Autodesk Inventor part; units mm, degrees
ref_plane "YZ Plane" through (0, 0, 0) normal (1, 0, 0) x (0, 1, 0)
ref_plane "XZ Plane" through (0, 0, 0) normal (0, 1, 0) x (-1, 0, 0)
ref_plane "XY Plane" through (0, 0, 0) normal (0, 0, 1) x (1, 0, 0)
ref_plane "Work Plane1" through (0, 0, 0) normal (0, 0, 1) x (1, 0, 0)
sketch "Sketch1" plane through (0, 0, 0) normal (0, 0, 1) x (1, 0, 0)
  circle A0 centre (23.85, -37.9212) radius 0.7
  circle A1 centre (23.85, -26.8413) radius 0.7
  circle A2 centre (10.55, -52.3871) radius 14
  circle A3 centre (10.55, -11.45) radius 14
  line L0 (25.25, -34.8579) -> (25.25, -62.5871)
  line L1 (22.15, -44.5487) -> (26.25, -44.5487)
  line L2 (26.25, -44.5487) -> (26.25, -19.2884)
  line L3 (26.25, -19.2884) -> (22.15, -19.2884)
  line L4 (22.15, -19.2884) -> (22.15, -44.5487)
  circle A4 centre (24.2, -42.4987) radius 2.05
  circle A5 centre (24.2, -21.3384) radius 2.05
  point P0 (0, 0)
  point P1 (24.2, -19.2884)
  point P2 (22.15, -21.3384)
  point P3 (22.15, -42.4987)
  point P4 (24.2, -44.5487)
  dimension "d0" = 1
  dimension "d1" = 1
extrude "Extrusion1" add sketch "Sketch1" along normal blind 3.5 contours A0 | A1 | A4 L0 L1 | A4 L0 | L4 A5 L2 A4 | L0 A4 L2 L1 | L0 A4 | A5 | L3 L2 A5
sketch "Sketch2" plane through (0, 0, 3.5) normal (0, 0, 1) x (1, 0, 0)
  line L0 (22.25, -33.4185) -> (19.55, -33.4185)
  line L1 (22.25, -30.4185) -> (19.55, -30.4185)
  line L2 (26.25, -33.9066) -> (26.25, -41.9871)
  line L3 (26.25, -29.1685) -> (26.25, -34.6685)
  line L4 (26.25, -21.85) -> (26.25, -29.9304)
  line L5 (22.15, -21.3384) -> (22.15, -42.4987)
  line L6 (26.25, -33.9185) -> (20.65, -33.9185)
  line L7 (20.65, -33.9185) -> (20.65, -29.9185)
  line L8 (20.65, -29.9185) -> (26.25, -29.9185)
  line L9 (26.25, -29.9185) -> (26.25, -33.9185)
  point P0 (0, 0)
  dimension "d4" = 0.5
  dimension "d5" = 0.5
  dimension "d6" = 1.5
extrude "Extrusion2" add sketch "Sketch2" along normal blind 5.5
sketch "Sketch3" plane through (20.65, -33.9185, 3.5) normal (0, -1, 0) x (1, 0, 0)
  circle A0 centre (-2.1, 3) radius 1.25
  line L0 (5.6, 0) -> (5.6, 5.5)
  circle A1 centre (2.4, 3) radius 1.25
  line L1 (2.4, 3) -> (-2.1, 3)
  circle A2 centre (2.4, 3) radius 2.5
  point P0 (-20.65, -3.5)
  dimension "d17" = 5
  dimension "d18" = 0.7
extrude "Extrusion3" cut sketch "Sketch3" against normal blind 11.5 contours A1
fillet "Fillet1" radius 2 2 edges at (20.65, -31.9185, 9) (20.65, -31.9185, 3.5)
ref_plane "Work Plane2" through (0, 0, 19.2) normal (0, 0, 1) x (1, 0, 0)
mirror "Mirror1" about plane through (0, 0, 19.2) normal (0, 0, 1) of "Extrusion1", "Extrusion2", "Extrusion3", "Fillet1"
sketch "Sketch4" plane through (0, 0, 3.5) normal (0, 0, 1) x (1, 0, 0)
  line L0 (26.25, -44.5487) -> (26.25, -19.2884)
  line L1 (24.2, -44.5487) -> (26.25, -44.5487)
  line L2 (26.25, -19.2884) -> (24.2, -19.2884)
  line L3 (25.75, -44.5487) -> (25.75, -19.2884)
  arc A0 (22.15, -42.4987) -> (24.2, -44.5487) centre (24.2, -42.4987) ccw
  line L4 (22.15, -21.3384) -> (22.15, -42.4987)
  arc A1 (24.2, -19.2884) -> (22.15, -21.3384) centre (24.2, -21.3384) ccw
  line L5 (25.75, -40.5487) -> (22.15, -40.5487)
  point P0 (0, 0)
  dimension "d14" = 0.5
  dimension "d20" = 4
extrude "Extrusion4" add sketch "Sketch4" along normal up to surface (31.4 mm away) contours L1 L3 L2 L0 | L1 A0 L4 L5 L3
fillet "Fillet2" radius 0.5 7 edges at (25.75, -37.2336, 3.5) (25.75, -24.6035, 3.5) (25.75, -37.2336, 34.9) (25.75, -24.6035, 34.9) (25.75, -40.5487, 19.2) (25.75, -31.9185, 9) (25.75, -31.9185, 29.4)
sketch "Sketch5" plane through (24.2, -19.2884, 38.4) normal (0, 0, 1) x (1, 0, 0)
  circle A0 centre (-0.35, -17.7307) radius 0.7
  circle A1 centre (-0.35, -6.4868) radius 0.7
  point P0 (-24.2, 19.2884)
hole "Hole1" at (23.85, -37.0191, 38.4) at (23.85, -25.7752, 38.4) direction (0, 0, -1) diameter 1.567 depth 6.3 countersink diameter 2 countersink angle 90
sketch "Sketch6" plane through (0, 0, 0) normal (0, 0, -1) x (-1, 0, 0)
  circle A0 centre (-23.85, -26.8413) radius 0.7
  circle A1 centre (-23.85, -37.9212) radius 0.7
  point P0 (0, 0)
hole "Hole2" at (23.85, -26.8413, 0) at (23.85, -37.9212, 0) direction (0, 0, 1) diameter 1.567 depth 6.3 countersink diameter 2 countersink angle 90
equation "\"d5\" = d4"
properties part number "DriverDownholdAlternate"
CAD build for the part. Positions are in the model's coordinates, mm. A direction names the side the tool comes from. Coordinates: 2 decimals unless noted, no trailing zeros. Order: outer loops, then holes, each group sorted by start corner. A loop starts at its lowest first (then second) coordinate and runs counter-clockwise, first axis right, second up. Notation, with made-up numbers: M 74,-9.5 L 129,-9.5 A24 cw 129,26.5 Z; hole C 9.5,52 d1. An arc over 180 degrees is marked long. Answer as CSV lines item,"result".
1) Cut at B-B (x = 21.05). List the corners of the cut face in (y, z), then the cut area to 3 significant figures.
Verdict:
outline,"M -33.92,4.24 L -29.92,4.24 L -29.92,8.2 L -33.92,8.2 Z; M -33.92,30.2 L -29.92,30.2 L -29.92,34.16 L -33.92,34.16 Z"
area,"31.7 mm2"
2) Cut at A-A (z = 31.9). List the corners of the cut face in (x, y), then the cut area to 3 significant figures.
Verdict:
outline,"M 20.65,-33.92 L 21.8,-33.92 L 21.8,-29.92 L 20.65,-29.92 Z; M 22.15,-42.5 A2.05 ccw 24.2,-44.55 L 26.25,-44.55 L 26.25,-19.29 L 25.75,-19.29 L 25.75,-29.92 L 24.3,-29.92 L 24.3,-33.92 L 25.75,-33.92 L 25.75,-40.05 A0.5 cw 25.25,-40.55 L 22.15,-40.55 Z"
area,"36.6 mm2"
3) Cut at C-C (y = -33). List the corners of the cut face in (x, z), then the cut area to 3 significant figures.
Verdict:
outline,"M 20.65,5.44 A2 ccw 22.15,3.5 L 22.15,0 L 26.25,0 L 26.25,38.4 L 22.15,38.4 L 22.15,34.9 A2 ccw 20.65,32.96 L 20.65,31.4 A2 ccw 22.65,29.4 L 25.25,29.4 A0.5 cw 25.75,28.9 L 25.75,9.5 A0.5 cw 25.25,9 L 22.65,9 A2 ccw 20.65,7 Z; hole C 23.05,6.5 d2.5; hole C 23.05,31.9 d2.5"
area,"87.6 mm2"
4) 3-axis set-ups, long thin cutter, end or side, ignore diameter. For faces 5 (the flat face through (23, -33.918, 5)), 6 (the cylindrical face through (22.06, -31.95, 5.74)), 7 (the flat face through (23.7, -24.5, 34.9)): which of +Z, -Z, +X, -X, +Y, -Y reach the whole face in a straight line?
Verdict:
face 5,"-X"
face 6,"+Y"
face 7,"-X, +Y"
5) Drill centre lines: L1, parallel to Z at x = 22.95, y = -33.75; L2, parallel to Y at x = 23.8, z = 35; L3, parallel to Z at x = 24, y = -24. Where is each one in solid material? Low to high. Write a range as from..to.
Verdict:
L1,"0..5.25, 7.75..9, 29.4..30.65, 33.15..38.4"
L2,"-44.51..-37.8, -36.24..-26.56, -24.99..-19.33"
L3,"0..3.5, 34.9..38.4"
6) Mould opens along X. For faces 1 (the flat face through (24, -32, 0)), 2 (the cylindrical face through (24.545, -26.48, 1.881)), 3 (the cylindrical face through (21.25, -31.95, 8.43)), 4 (the cylindrical face through (24.15, -37.743, 36.519)) say: released by +X, released by -X, zero draft, split by the parting line, or undercut.
Verdict:
face 1,"zero draft"
face 2,"undercut"
face 3,"released by -X"
face 4,"undercut"
7) Cut at D-D (z = 26.5). List the corners of the cut face in (x, y).
Verdict:
outline,"M 22.15,-42.5 A2.05 ccw 24.2,-44.55 L 26.25,-44.55 L 26.25,-19.29 L 25.75,-19.29 L 25.75,-40.05 A0.5 cw 25.25,-40.55 L 22.15,-40.55 Z"
8) Flat gauge pins, fed straight in: P1, Ø6, axis at y = -29.5, z = 19, coming from the -X side; P2, Ø3, axis at x = 23.05, z = 31.9, coming from the +Y side; P3, Ø0.8, axis at x = 24, y = -31, coming from the -Z side; P4, Ø6.5, axis at y = -37, z = 13, coming from the -X side. Where does each tip first touch, or does it go through?
Verdict:
P1,"x = 25.75"
P2,"y = -29.92"
P3,"z = 0"
P4,"x = 25.71"
